```python
from build123d import *

# Parameters (mm, degrees)
SKETCH1_W               = 60
SKETCH1_H               = 10
BOSS_EXTRUDE1_DEPTH     = 4
SKETCH2_R               = 1.75
CUT_EXTRUDE1_DEPTH      = 4
SKETCH3_W               = 10
SKETCH3_H               = 4
BOSS_EXTRUDE2_DEPTH     = 40
SKETCH4_R               = 1.5
CUT_EXTRUDE2_DEPTH      = 10
CUT_EXTRUDE3_DEPTH      = 71.823724839
CUT_EXTRUDE3_DEPTH_BACK = 71.823724839
SKETCH5_W               = 6
SKETCH5_H               = 4
FILLET1_R               = 1


with BuildPart() as part:
    # Sketch1 → Boss-Extrude1 (new body)
    with BuildSketch(Plane(origin=(0, 0, 0), x_dir=(1, 0, 0), z_dir=(0, 1, 0))):
        Rectangle(SKETCH1_W, SKETCH1_H)
    extrude(amount=BOSS_EXTRUDE1_DEPTH)

    # Sketch2 → Cut-Extrude1 (cut)
    with BuildSketch(Plane(origin=(0, 4, 0), x_dir=(1, 0, 0), z_dir=(0, 1, 0))):
        with Locations(Location((-26, 0, 0), (0, 0, 270))):
            Circle(SKETCH2_R)
        with Locations(Location((7.5, 0, 0), (0, 0, 270))):
            Circle(SKETCH2_R)
        with Locations(Location((25, 0, 0), (0, 0, 270))):
            Circle(SKETCH2_R)
        with Locations(Location((-15, 0, 0), (0, 0, 270))):
            Circle(SKETCH2_R)
    extrude(amount=-CUT_EXTRUDE1_DEPTH, mode=Mode.SUBTRACT)

    # Sketch3 → Boss-Extrude2 (add)
    with BuildSketch(Plane(origin=(30, 0, 0), x_dir=(0, 0, -1), z_dir=(1, 0, 0))):
        with Locations((0, 2)):
            Rectangle(SKETCH3_W, SKETCH3_H)
    extrude(amount=BOSS_EXTRUDE2_DEPTH)

    # Sketch4 → Cut-Extrude2 (cut)
    with BuildSketch(Plane(origin=(0, 4, 0), x_dir=(1, 0, 0), z_dir=(0, 1, 0))):
        with Locations(Location((59.32, 0, 0), (0, 0, 270))):
            Circle(SKETCH4_R)
    extrude(amount=-CUT_EXTRUDE2_DEPTH, mode=Mode.SUBTRACT)

    # Sketch5 → Cut-Extrude3 (cut, two sides: drawn at the far end of the back side and taken through both)
    with BuildSketch(Plane.XY.offset(5).offset(-CUT_EXTRUDE3_DEPTH_BACK)):
        with Locations((67, 2)):
            Rectangle(SKETCH5_W, SKETCH5_H)
    extrude(amount=CUT_EXTRUDE3_DEPTH + CUT_EXTRUDE3_DEPTH_BACK, mode=Mode.SUBTRACT)

    # Fillet1
    fillet1_edges = [part.edges().sort_by_distance(p)[0] for p in [
        (-30, 4, 0),
        (17, 4, 5),
        (17, 0, 5),
        (17, 0, -5),
        (17, 4, -5),
        (-30, 0, 0),
        (64, 0, 0),
        (64, 2, 5),
        (64, 2, -5),
        (64, 4, 0),
        (-30, 2, 5),
        (-30, 2, -5),
    ]]
    fillet(fillet1_edges, radius=FILLET1_R)


solid = part.part
```
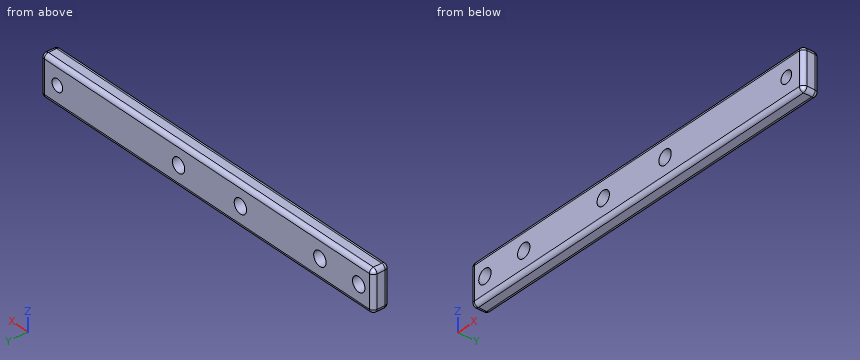
Could you check a few things on this model? Use its own coordinates, in mm. Round coordinates to 2 decimals unless told otherwise and drop trailing zeros. Loops run counter-clockwise (first coordinate to the right, second up) from the corner with the lowest first, then second, coordinate; pieces in that order, holes last.
Q1. I want a section at A-A (z = 0). Write out the boundary of the cut face in (x, y), and give its area (3 significant figures).
Q2. I want a section at D-D (x = 49.5). Write out the boundary of the cut face in (y, z), and give its area (3 significant figures).
Q3. For P1, Ø2, axis at x = -26, z = 0, coming from the -Y side; P2, Ø2, axis at y = 0.5, z = -1.5, coming from the +X side, each with a flat end and sliding along its axis, tell me the tip position at first contact or that it passes through.
Q4. Please list where these lines run through material, in increasing order: L1, parallel to X at y = 1.6, z = 0; L2, parallel to Z at x = -16.5, y = 1.8; L3, parallel to Y at x = 31, z = -4.5.
Q5. I want a section at C-C (x = -26). Write out the boundary of the cut face in (y, z).
Q6. I want a section at B-B (y = 1.85). Write out the boundary of the cut face in (x, z).
Answer below:
1. outline: (-30, 1) arc R1 ccw to (-29, 0) - (-27.75, 0) - (-27.75, 4) - (-29, 4) arc R1 ccw to (-30, 3) - close; (-24.25, 0) - (-16.75, 0) - (-16.75, 4) - (-24.25, 4) - close; (-13.25, 0) - (5.75, 0) - (5.75, 4) - (-13.25, 4) - close; (9.25, 0) - (23.25, 0) - (23.25, 4) - (9.25, 4) - close; (26.75, 0) - (57.82, 0) - (57.82, 4) - (26.75, 4) - close; (60.82, 0) - (63, 0) arc R1 ccw to (64, 1) - (64, 3) arc R1 ccw to (63, 4) - (60.82, 4) - close
1. area: 307 mm2
2. outline: (0, -4) arc R1 ccw to (1, -5) - (3, -5) arc R1 ccw to (4, -4) - (4, 4) arc R1 ccw to (3, 5) - (1, 5) arc R1 ccw to (0, 4) - close
2. area: 39.1 mm2
3. P1: passes through
3. P2: stops at x = 64
4. L1: x = -30 to -27.75, -24.25 to -16.75, -13.25 to 5.75, 9.25 to 23.25, 26.75 to 57.82, 60.82 to 64
4. L2: z = -5 to -0.9, 0.9 to 5
4. L3: y = 0.13 to 3.87
5. outline: (0, -4) arc R1 ccw to (1, -5) - (3, -5) arc R1 ccw to (4, -4) - (4, -1.75) - (0, -1.75) - close; (0, 1.75) - (4, 1.75) - (4, 4) arc R1 ccw to (3, 5) - (1, 5) arc R1 ccw to (0, 4) - close
6. outline: (-30, -4) arc R1 ccw to (-29, -5) - (63, -5) arc R1 ccw to (64, -4) - (64, 4) arc R1 ccw to (63, 5) - (-29, 5) arc R1 ccw to (-30, 4) - close; hole circle Ø3.5 at (-26, 0); hole circle Ø3.5 at (-15, 0); hole circle Ø3.5 at (7.5, 0); hole circle Ø3.5 at (25, 0); hole circle Ø3 at (59.32, 0)
